Verification items for this drawing (mm, ordinates from the low corner). A direction names the side the tool comes from. Coordinates: 2 decimals unless noted, no trailing zeros. Loops run counter-clockwise (first coordinate to the right, second up) from the corner with the lowest first, then second, coordinate; pieces in that order, holes last. Notation, with made-up numbers: (10, -31) -> (15, -31) arc R14 ccw to (15, -18) -> close; hole circle Ø2 at (22, 87). An arc over 180 degrees is marked (long way). Write item = value, one per line.
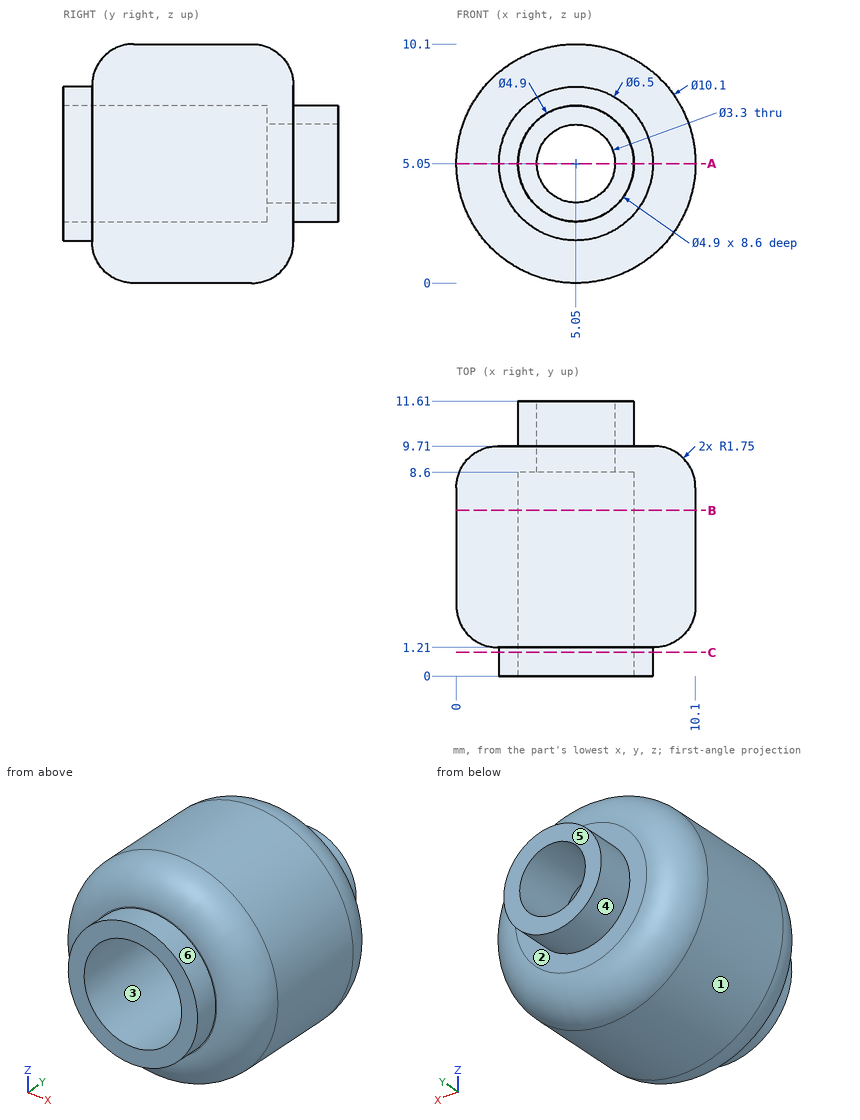
1) Sectioned sample at B-B, the plane y = 7. Record the cut outline in (x, z).
Ans:
outline = circle Ø10.1 at (5.05, 5.05); hole circle Ø4.9 at (5.05, 5.05)
2) Sectioned sample at A-A, the plane z = 5.05. Record the cut outline in (x, y).
Ans:
outline = (0, 2.96) arc R1.75 ccw to (1.75, 1.21) -> (1.8, 1.21) -> (1.8, 0) -> (2.6, 0) -> (2.6, 8.6) -> (3.4, 8.6) -> (3.4, 11.61) -> (2.6, 11.61) -> (2.6, 9.71) -> (1.75, 9.71) arc R1.75 ccw to (0, 7.96) -> close; (6.7, 8.6) -> (7.5, 8.6) -> (7.5, 0) -> (8.3, 0) -> (8.3, 1.21) -> (8.35, 1.21) arc R1.75 ccw to (10.1, 2.96) -> (10.1, 7.96) arc R1.75 ccw to (8.35, 9.71) -> (7.5, 9.71) -> (7.5, 11.61) -> (6.7, 11.61) -> close
3) Release check for a two-part mould opening along Z. For the marked faces 1, 2 and 3 record: pulls with the +Z half, pulls with the -Z half, needs draft (parallel to the pull), parting line crosses it, or undercut.
Ans:
face_1 = parting line crosses it
face_2 = needs draft
face_3 = undercut
4) Depth check by flat-ended pin: pin 1 Ø2 at (x, z) = (6, 3.5) entering from -Y; pin 2 Ø2 at (y, z) = (2.5, 3.5) entering from -X; pin 3 Ø4 at (x, z) = (5.05, 5.05) entering from -Y; pin 4 Ø3 at (x, z) = (1.5, 1.5) entering from +Y. Enter the tip coordinate at first touch or a pass-through.
Ans:
pin_1 = 0
pin_2 = 0.04
pin_3 = 8.6
pin_4 = 9.7
5) Tool access check on the marked faces 4, 5 and 6. Record the directions out of +Z, -Z, +X, -X, +Y, -Y that give a thin tool (end or side, any length) a straight path to the whole face; none if there is none.
Ans:
face_4 = +Y
face_5 = +Z, -Z, +X, -X, +Y
face_6 = -Y
6) Material ranges on line 1 (X direction, y = 3.5, z = 5.05); line 2 (X direction, y = 10.35, z = 5.05); line 3 (Y direction, x = 8, z = 6.75), recorded low to high.
Ans:
line_1 = 0 to 2.6, 7.5 to 10.1
line_2 = 2.6 to 3.4, 6.7 to 7.5
line_3 = 1.21 to 9.71
7) Sectioned sample at C-C, the plane y = 1. Record the cut outline in (x, z), plus the area to 3 significant figures.
Ans:
outline = circle Ø6.5 at (5.05, 5.05); hole circle Ø4.9 at (5.05, 5.05)
area = 14.3 mm2
